Verification items for the finished model (mm, model axes). Face numbers are marked on the shaded views. A direction names the side the tool comes from. Round coordinates to 2 decimals unless told otherwise and drop trailing zeros. Order: outer loops, then holes, each group sorted by start corner. A loop starts at its lowest first (then second) coordinate and runs counter-clockwise, first axis right, second up. Notation, with made-up numbers: M 8.25,28 L 32.25,28 A23 ccw 32.25,67 Z; hole C 76.25,12 d10. An arc over 180 degrees is marked long. Answer as a JSON object with one key per item and string values. Group by question number.
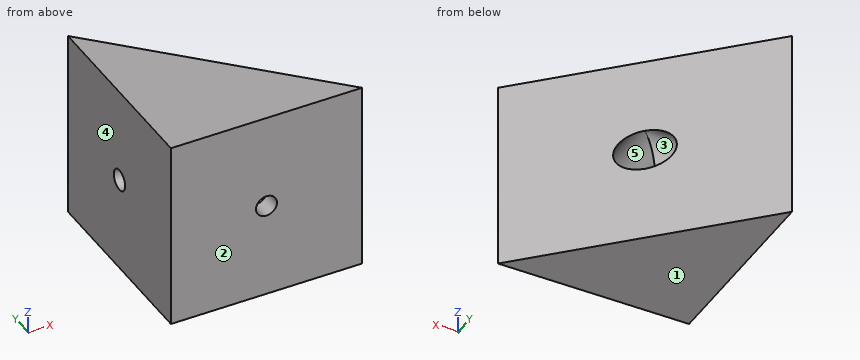
```python
from build123d import *

# Parameters (mm, degrees)
F2_DEPTH  = 30
F4_R      = 3.25
F5_DEPTH  = 27.001
F6_R      = 1.65
F7_DEPTH  = 3.001
F9_R      = 3.25
F10_DEPTH = 27.001
F11_R     = 1.65
F12_DEPTH = 25


with BuildPart() as f2:
    # F1 (on Top) → F2 (new body)
    with BuildSketch(Plane.XY):
        Polygon((-15, -15), (15, -15), (-15, 15), align=None)
    extrude(amount=F2_DEPTH)

    # F4 (on offset) → F5 (cut, through all)
    with BuildSketch(Plane(origin=(-12, 0, 0), x_dir=(0, -1, 0), z_dir=(-1, 0, 0))):
        with Locations((0, 15)):
            Circle(F4_R)
    extrude(amount=-F5_DEPTH, mode=Mode.SUBTRACT)

    # F6 (on offset) → F7 (cut, through all)
    with BuildSketch(Plane(origin=(-12, 0, 0), x_dir=(0, -1, 0), z_dir=(-1, 0, 0))):
        with Locations((0, 15)):
            Circle(F6_R)
    extrude(amount=F7_DEPTH, mode=Mode.SUBTRACT)

    # F9 (on offset) → F10 (cut, through all)
    with BuildSketch(Plane.XZ.offset(12)):
        with Locations((0, 15)):
            Circle(F9_R)
    extrude(amount=-F10_DEPTH, mode=Mode.SUBTRACT)

    # F11 (on offset) → F12 (cut)
    with BuildSketch(Plane.XZ.offset(12)):
        with Locations((0, 15)):
            Circle(F11_R)
    extrude(amount=F12_DEPTH, mode=Mode.SUBTRACT)


solid = f2.part
```
Q1. Release check for a two-part mould opening along Z. For the marked faces 1, 2 and 3 record: released by +Z, released by -Z, zero draft, split by the parting line, or undercut.
Q2. Cross-section at B-B, the plane y = -4.5. Record the cut outline in (x, z), then the cut area to 3 significant figures.
Q3. Cross-section at A-A, the plane z = 15. Record the cut outline in (x, y), then the cut area to 3 significant figures.
Q4. Tool access check on the marked faces 4 and 5. Record the directions out of +Z, -Z, +X, -X, +Y, -Y that give a thin tool (end or side, any length) a straight path to the whole face; none if there is none.
Q5. Gauge pin test, flat ends, axial feed: pin 1 Ø3 at (y, z) = (0.5, 14) entering from +X; pin 2 Ø7.5 at (x, z) = (0, 15) entering from +Y; pin 3 Ø2 at (x, z) = (-0.5, 15.5) entering from +Y; pin 4 Ø2.5 at (x, z) = (0, 15) entering from +Y. Record the tip position at first contact, or that the pin passes through.
Q6. Cross-section at C-C, the plane y = 12. Record the cut outline in (x, z).
Q7. Cross-section at D-D, the plane z = 27. Record the cut outline in (x, y).
Q8. Thickness scan on line 1 (Z direction, x = 0, y = -12.75); line 2 (Z direction, x = 0, y = -7.5); line 3 (Y direction, x = 0, z = 22.75). Record the ranges inside material, lowest first. Write a range as from..to.
Conclusion:
{
 "1": {"face 1": "released by -Z", "face 2": "zero draft", "face 3": "undercut"},
 "2": {"outline": "M -15,0 L 4.5,0 L 4.5,30 L -15,30 Z; hole C 0,15 d6.5", "area": "552 mm2"},
 "3": {"outline": "M -15,-15 L -1.65,-15 L -1.65,-12 L -3.25,-12 L -3.25,-3.25 L -12,-3.25 L -12,-1.65 L -15,-1.65 Z; M -15,1.65 L -12,1.65 L -12,3.25 L -3.25,3.25 L -15,15 Z; M 1.65,-15 L 15,-15 L 3.25,-3.25 L 3.25,-12 L 1.65,-12 Z", "area": "295 mm2"},
 "4": {"face 4": "+Z, -Z, -X, +Y, -Y", "face 5": "+Y"},
 "5": {"pin 1": "x = -12", "pin 2": "y = 3.75", "pin 3": "y = -12", "pin 4": "through"},
 "6": {"outline": "M -15,0 L -12,0 L -12,30 L -15,30 Z"},
 "7": {"outline": "M -15,-15 L 15,-15 L -15,15 Z"},
 "8": {"line 1": "0..13.35, 16.65..30", "line 2": "0..11.75, 18.25..30", "line 3": "-15..0"}
}
